```python
from build123d import *

# Parameters (mm, degrees)
SKETCH1_W               = 320
SKETCH1_H               = 30
BOSS_EXTRUDE1_DEPTH     = 25
SKETCH2_W               = 280
SKETCH2_H               = 30
CUT_EXTRUDE1_DEPTH      = 25
CUT_EXTRUDE3_DEPTH      = 163.634559673
CUT_EXTRUDE3_DEPTH_BACK = 163.634559673
SKETCH3_R               = 5


with BuildPart() as part:
    # Sketch1 → Boss-Extrude1 (new, symmetric)
    with BuildSketch(Plane.XY):
        Rectangle(SKETCH1_W, SKETCH1_H)
    extrude(amount=BOSS_EXTRUDE1_DEPTH, both=True)

    # Sketch2 → Cut-Extrude1 (cut, symmetric)
    with BuildSketch(Plane(origin=(0, 0, 0), x_dir=(1, 0, 0), z_dir=(0, 1, 0))):
        Rectangle(SKETCH2_W, SKETCH2_H)
    extrude(amount=CUT_EXTRUDE1_DEPTH, both=True, mode=Mode.SUBTRACT)

    # Sketch3 → Cut-Extrude3 (cut, two sides: drawn at the far end of the back side and taken through both)
    with BuildSketch(Plane.XY.offset(-CUT_EXTRUDE3_DEPTH_BACK)):
        with Locations((-150, 0)):
            Circle(SKETCH3_R)
        with Locations((150, 0)):
            Circle(SKETCH3_R)
        with Locations((-50, 0)):
            Circle(SKETCH3_R)
        with Locations((50, 0)):
            Circle(SKETCH3_R)
    extrude(amount=CUT_EXTRUDE3_DEPTH + CUT_EXTRUDE3_DEPTH_BACK, mode=Mode.SUBTRACT)


solid = part.part
```
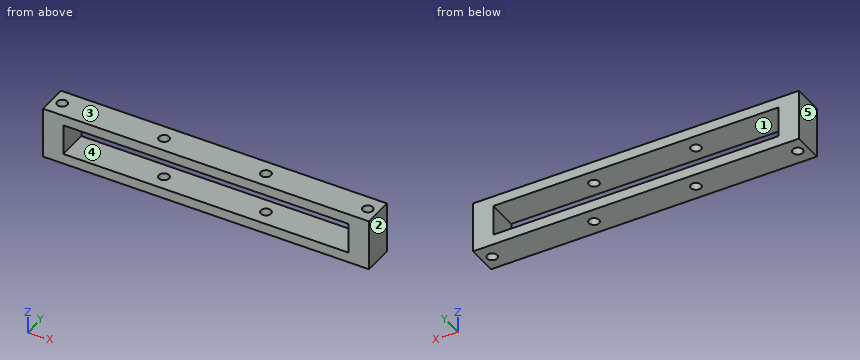
The listing builds one solid part. Answer for the finished solid, in the listing's coordinates (mm). Face numbers are marked on the shaded views. A direction names the side the tool comes from. Round coordinates to 2 decimals unless told otherwise and drop trailing zeros. Order: outer loops, then holes, each group sorted by start corner. A loop starts at its lowest first (then second) coordinate and runs counter-clockwise, first axis right, second up. Notation, with made-up numbers: (-23.75, 64) - (-16.75, 64) arc R33 cw to (-16.75, 98) - close; hole circle Ø10 at (84.25, 14). An arc over 180 degrees is marked (long way). Put each result on its own line as item: value. Start each with the question number.
(1) For the marked faces 4 and 5, determine the directions among +Z, -Z, +X, -X, +Y, -Y from which every point of the face is accessible in a straight line to the end or side of a thin tool.
(2) Straight lines are drawn through the part: probe 1 along X at (y, z) = (0.75, -22); probe 2 along X at (y, z) = (0, -19); probe 3 along Z at (x, y) = (-68.5, -0.25). For each, find the intervals that lie inside material, in ascending order. Write a range as from..to.
(3) Find section A-A (z = -8). Give the vertices of the cut face in (x, y).
(4) Determine the mould class of the marked faces 1, 2 and 3 for opening direction X: released by +X, released by -X, zero draft, split by the parting line, or undercut.
(5) Find section D-D (z = 19). Give the vertices of the cut face in (x, y), plus the area to 3 significant figures.
(6) Find section C-C (y = -12). Give the vertices of the cut face in (x, z), plus the area to 3 significant figures.
(7) Find section B-B (x = 50). Give the vertices of the cut face in (y, z), plus the area to 3 significant figures.
Reply:
1. face 4: +Y, -Y
1. face 5: +Z, -Z, -X, +Y, -Y
2. probe 1: -160..-154.94, -145.06..-54.94, -45.06..45.06, 54.94..145.06, 154.94..160
2. probe 2: -160..-155, -145..-55, -45..45, 55..145, 155..160
2. probe 3: -25..-15, 15..25
3. outline: (-160, -15) - (-140, -15) - (-140, 15) - (-160, 15) - close; (140, -15) - (160, -15) - (160, 15) - (140, 15) - close; hole circle Ø10 at (-150, 0); hole circle Ø10 at (150, 0)
4. face 1: undercut
4. face 2: released by +X
4. face 3: zero draft
5. outline: (-160, -15) - (160, -15) - (160, 15) - (-160, 15) - close; hole circle Ø10 at (-150, 0); hole circle Ø10 at (-50, 0); hole circle Ø10 at (50, 0); hole circle Ø10 at (150, 0)
5. area: 9,290 mm^2
6. outline: (-160, -25) - (160, -25) - (160, 25) - (-160, 25) - close; hole (-140, -15) - (140, -15) - (140, 15) - (-140, 15) - close
6. area: 7,600 mm^2
7. outline: (-15, -25) - (-5, -25) - (-5, -15) - (-15, -15) - close; (-15, 15) - (-5, 15) - (-5, 25) - (-15, 25) - close; (5, -25) - (15, -25) - (15, -15) - (5, -15) - close; (5, 15) - (15, 15) - (15, 25) - (5, 25) - close
7. area: 400 mm^2
